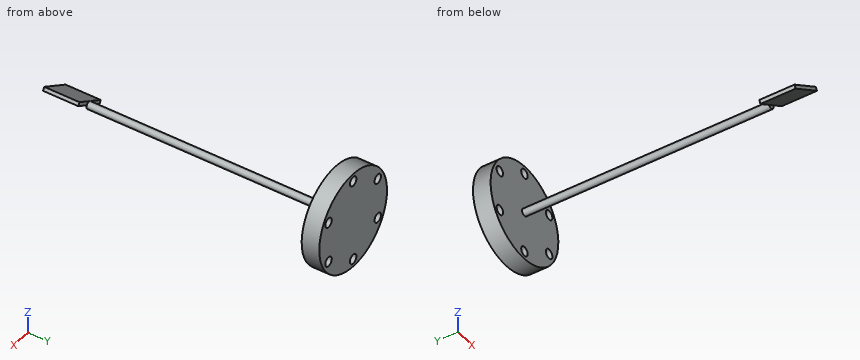
```python
from build123d import *

# Parameters (mm, degrees)
SKETCH1_R           = 34.925
EXTRUDE1_DEPTH      = 12.7
SKETCH3_R           = 3.3655
CUT_EXTRUDE2_DEPTH  = 12.7
CIRPATTERN1_COUNT   = 6
SKETCH8_R           = 2.54
EXTRUDE3_DEPTH      = 177.8
EXTRUDE_THIN1_DEPTH = 25.4


with BuildPart() as part:
    # Sketch1 → Extrude1 (new body)
    with BuildSketch(Plane(origin=(0, 0, 0), x_dir=(1, 0, 0), z_dir=(0, 1, 0))):
        with Locations(Location((0, 0, 0), (0, 0, 270))):
            Circle(SKETCH1_R)
    extrude(amount=EXTRUDE1_DEPTH)

    # Sketch3 → Cut-Extrude2 (cut)
    with BuildSketch(Plane(origin=(0, 0, 0), x_dir=(1, 0, 0), z_dir=(0, 1, 0))):
        with Locations(Location((0, 29.337, 0), (0, 0, 270))):
            Circle(SKETCH3_R)
    cut_extrude2 = extrude(amount=CUT_EXTRUDE2_DEPTH, mode=Mode.SUBTRACT)

    # CirPattern1: Cut-Extrude2 ×6 about axis
    cirpattern1_axis = Axis((0, 0, 0), (0, 1, 0))
    for i in range(1, CIRPATTERN1_COUNT):
        add(cut_extrude2.rotate(cirpattern1_axis, i * 360 / CIRPATTERN1_COUNT), mode=Mode.SUBTRACT)

    # Sketch8 → Extrude3 (add)
    with BuildSketch(Plane.XZ):
        with Locations(Location((0, 0, 0), (0, 0, 90))):
            Circle(SKETCH8_R)
    extrude(amount=EXTRUDE3_DEPTH)

    # Sketch12 → Extrude-Thin1 (add)
    with BuildSketch(Plane.XZ.offset(177.8)):
        Polygon((10.998522628, 6.35), (0, 0), (-10.998522628, -6.35), (-12.268522628, -4.150295474), (-1.27, 2.199704526), (9.728522628, 8.549704526), align=None)
    extrude(amount=EXTRUDE_THIN1_DEPTH)


solid = part.part
```
Here's how the part is built. I have some questions about the finished solid (model axes, mm). Coordinates: 2 decimals unless noted, no trailing zeros. Write each loop counter-clockwise with the first axis right and the second up, starting at its lowest first coordinate (ties: lowest second). Pieces come first, ordered by that corner, then holes. Notation, with made-up numbers: M -23,11 L 17,11 A13 cw 17,18 Z; hole C 65,53.25 d7. An arc over 180 degrees is marked long. Answer as CSV lines item,"result". Start each with the question number.
Q1. Will these pins go through, and if not, where does the flat tip stop? pin 1 Ø3 at (x, z) = (0, -1) entering from -Y; pin 2 Ø12 at (x, y) = (5, -141) entering from +Z; pin 3 Ø11 at (x, z) = (-25.41, -14.67) entering from -Y.
Q2. Suppose I cut it at C-C, the plane x = 14.5. List the corners of the cut face in (y, z) for me, then the cut area to 3 significant figures.
Q3. Suppose I cut it at A-A, the plane x = 26.5. List the corners of the cut face in (y, z) for me, then the cut area to 3 significant figures.
Q4. Suppose I cut it at B-B, the plane y = -149. List the corners of the cut face in (x, z) for me.
Q5. I need wall thicknesses on probe 1 along Y at (x, z) = (13, -0.5); probe 2 along X at (y, z) = (-19.5, -1); probe 3 along Y at (x, z) = (1.5, -1). Which ranges of each line are inside material? Lowest first, please. Write a range as [from, to].
Entries:
1,pin 1,"stops at y = -203.2"
1,pin 2,"stops at z = 2.54"
1,pin 3,"stops at y = 0"
2,outline,"M 0,-31.77 L 12.7,-31.77 L 12.7,31.77 L 0,31.77 Z"
2,area,"807 mm²"
3,outline,"M 0,-22.75 L 12.7,-22.75 L 12.7,-17.85 L 0,-17.85 Z; M 0,-11.49 L 12.7,-11.49 L 12.7,11.49 L 0,11.49 Z; M 0,17.85 L 12.7,17.85 L 12.7,22.75 L 0,22.75 Z"
3,area,"416 mm²"
4,outline,"C 0,0 d5.08"
5,probe 1,"y = [0, 12.7]"
5,probe 2,"x = [-2.33, 2.33]"
5,probe 3,"y = [-177.8, 12.7]"
